Can you work these out from the drawing? Everything is in mm from the part's minimum corner. A direction names the side the tool comes from. Coordinates: 2 decimals unless noted, no trailing zeros. Order: outer loops, then holes, each group sorted by start corner. A loop starts at its lowest first (then second) coordinate and runs counter-clockwise, first axis right, second up. Notation, with made-up numbers: M -36.75,62.25 L -5.75,62.25 A20 cw -5.75,82.25 Z; hole C -18,68.5 d3. An arc over 180 degrees is marked long. One line per question, with ' | ' between items. Start each with the question number.
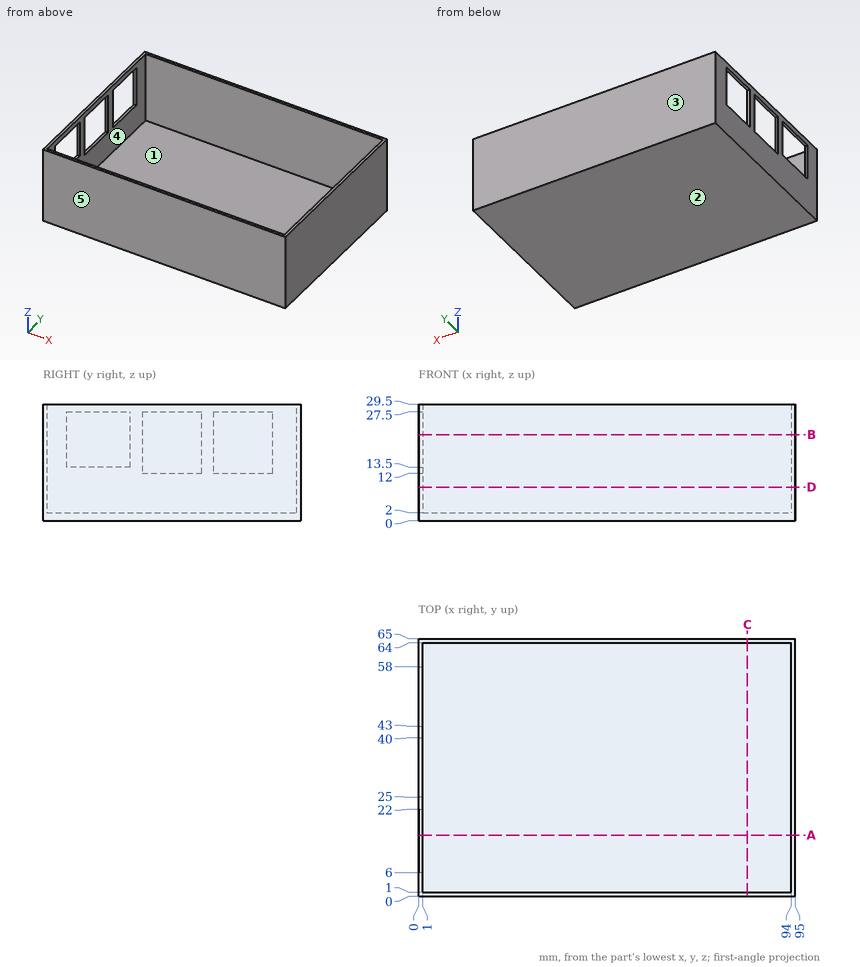
(1) Imagine slicing it at A-A, the plane y = 15.5. Write out the boundary of the cut face in (x, z).
(2) Imagine slicing it at C-C, the plane x = 83. Write out the boundary of the cut face in (y, z), plus the area to 3 significant figures.
(3) For P1, Ø4, axis at x = 14, y = 14, coming from the +Z side; P2, Ø0.8, axis at x = 0.5, z = 21.5, coming from the -Y side, each with a flat end and sliding along its axis, tell me the tip position at first contact or that it passes through.
(4) On a 3-axis mill with a long thin cutter (end or side, diameter ignored), from which of +Z, -Z, +X, -X, +Y, -Y can I reach the whole of each face in a straight line? I mean the marked faces 4 and 5. Say none if no direction works.
(5) Imagine slicing it at B-B, the plane z = 21.75. Write out the boundary of the cut face in (x, y).
(6) If I drill on line 1 along Y through (x, z) = (40, 28); line 2 along X through (y, z) = (57, 4.75); line 3 along Z through (x, y) = (56, 38.5), over which ranges is the centre line in solid material (lowest first)? Write a range as from..to.
(7) Imagine slicing it at D-D, the plane z = 8.5. Write out the boundary of the cut face in (x, y), plus the area to 3 significant figures.
(8) We'd pull the mould along Y, two halves only. Please class the marked faces 1, 2 and 3: +Y half, -Y half, draft (parallel to the pull), parting line (faces both ways), or undercut.
Answers:
1) outline: M 0,0 L 95,0 L 95,29.5 L 94,29.5 L 94,2 L 1,2 L 1,13.5 L 0,13.5 Z; M 0,27.5 L 1,27.5 L 1,29.5 L 0,29.5 Z
2) outline: M 0,0 L 65,0 L 65,29.5 L 64,29.5 L 64,2 L 1,2 L 1,29.5 L 0,29.5 Z | area: 185 mm²
3) P1: z = 2 | P2: y = 0
4) face 4: +Z | face 5: +Z, -Z, +X, -X, -Y
5) outline: M 0,0 L 95,0 L 95,65 L 0,65 L 0,58 L 1,58 L 1,64 L 94,64 L 94,1 L 1,1 L 1,6 L 0,6 Z; M 0,22 L 1,22 L 1,25 L 0,25 Z; M 0,40 L 1,40 L 1,43 L 0,43 Z
6) line 1: 0..1, 64..65 | line 2: 0..1, 94..95 | line 3: 0..2
7) outline: M 0,0 L 95,0 L 95,65 L 0,65 Z; hole M 1,1 L 94,1 L 94,64 L 1,64 Z | area: 316 mm²
8) face 1: undercut | face 2: draft | face 3: +Y half
